Could you check a few things on this drawing? It's one solid part, dimensions in mm from its lowest x, y, z. A direction names the side the tool comes from. Give positions to 0.01 mm unless a question says otherwise; leave off trailing zeros. Order: outer loops, then holes, each group sorted by start corner. A loop starts at its lowest first (then second) coordinate and runs counter-clockwise, first axis right, second up. Notation, with made-up numbers: (39.5, -30.75) - (80.5, -30.75) arc R22 ccw to (80.5, -3.75) - close; hole circle Ø6 at (-30, -16.5). An arc over 180 degrees is marked (long way). Return JSON: item names as keys, results as strings.
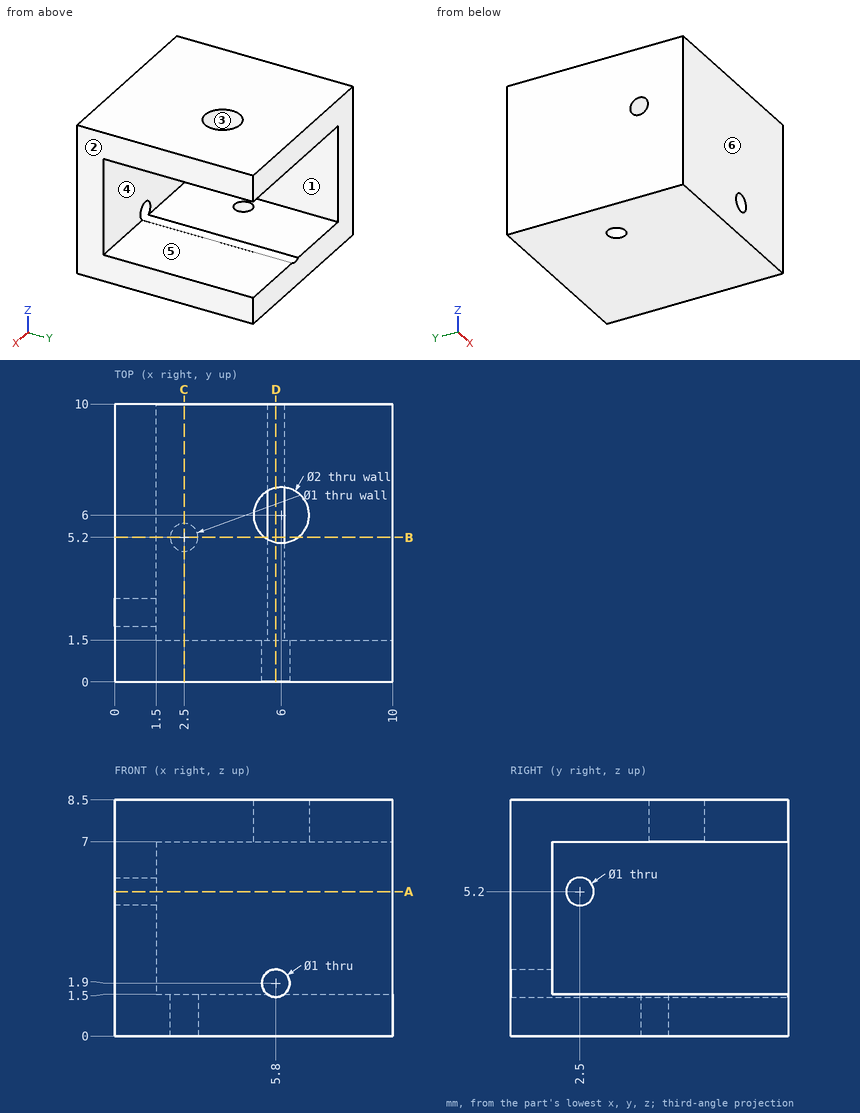
1. Suppose I cut it at B-B (y = 5.2). List the corners of the cut face in (x, z) for me, plus the area to 3 significant figures.
Checks:
{"outline": "(0, 0) - (2, 0) - (2, 1.5) - (1.5, 1.5) - (1.5, 7) - (5.4, 7) - (5.4, 8.5) - (0, 8.5) - close; (3, 0) - (10, 0) - (10, 1.5) - (6.1, 1.5) arc R0.5 cw to (5.5, 1.5) - (3, 1.5) - close; (6.6, 7) - (10, 7) - (10, 8.5) - (6.6, 8.5) - close", "area": "34.9 mm^2"}
2. Suppose I cut it at D-D (x = 5.8). List the corners of the cut face in (y, z) for me.
Checks:
{"outline": "(0, 0) - (10, 0) - (10, 1.4) - (0, 1.4) - close; (0, 2.4) - (1.5, 2.4) - (1.5, 7) - (5.02, 7) - (5.02, 8.5) - (0, 8.5) - close; (6.98, 7) - (10, 7) - (10, 8.5) - (6.98, 8.5) - close"}
3. Suppose I cut it at C-C (x = 2.5). List the corners of the cut face in (y, z) for me, plus the area to 4 significant figures.
Checks:
{"outline": "(0, 0) - (4.7, 0) - (4.7, 1.5) - (1.5, 1.5) - (1.5, 7) - (10, 7) - (10, 8.5) - (0, 8.5) - close; (5.7, 0) - (10, 0) - (10, 1.5) - (5.7, 1.5) - close", "area": "36.75 mm^2"}
4. On a 3-axis mill with a long thin cutter (end or side, diameter ignored), from which of +Z, -Z, +X, -X, +Y, -Y can I reach the whole of each face in a straight line? I mean the marked faces 1 and 2. Say none if no direction works.
Checks:
{"face 1": "+X, +Y", "face 2": "+Z, -Z, +X, +Y, -Y"}
5. For pin 1 Ø1.2 at (x, y) = (6, 6) entering from +Z, with a flat end and sliding along its axis, tell me the tip position at first contact or that it passes through.
Checks:
{"pin 1": "z = 1.5"}
6. Suppose I cut it at A-A (z = 5.2). List the corners of the cut face in (x, y) for me, plus the area to 4 significant figures.
Checks:
{"outline": "(0, 0) - (10, 0) - (10, 1.5) - (1.5, 1.5) - (1.5, 2) - (0, 2) - close; (0, 3) - (1.5, 3) - (1.5, 10) - (0, 10) - close", "area": "26.25 mm^2"}
7. If I drill on L1, parallel to Y at x = 0.4, z = 5.2; L2, parallel to Z at x = 3.5, y = 9.75; L3, parallel to Y at x = 2.5, z = 0.7, over which ranges is the centre line in solid material (lowest first)? Write a range as [from, to].
Checks:
{"L1": "[0, 2], [3, 10]", "L2": "[0, 1.5], [7, 8.5]", "L3": "[0, 4.7], [5.7, 10]"}
8. Thinking about a two-plate mould opening in Y: for the marked faces 3, 4, 5 and 6, which applies, +Y half, -Y half, draft (parallel to the pull), parting line (faces both ways), or undercut?
Checks:
{"face 3": "undercut", "face 4": "+Y half", "face 5": "draft", "face 6": "-Y half"}
